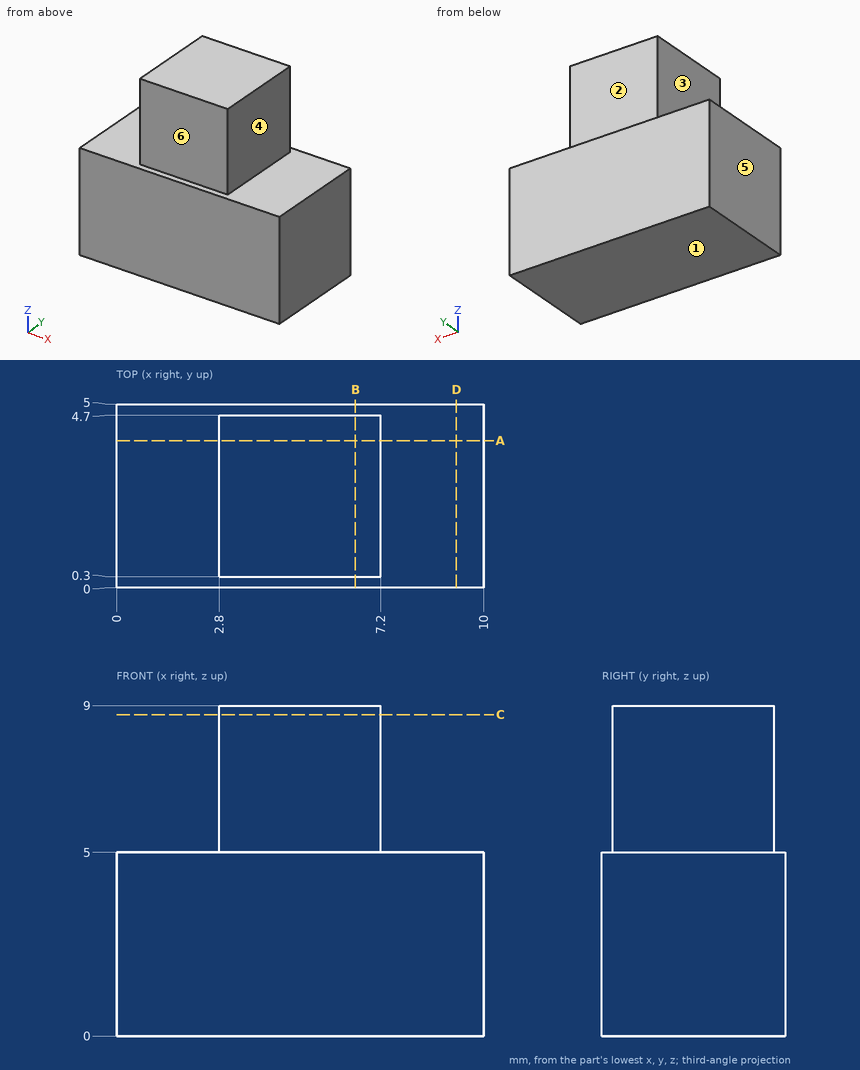
Geometry check sheet. Reference: drawing and pictorial views, mm from the part's lowest x, y, z. A direction names the side the tool comes from. Coordinates: 2 decimals unless noted, no trailing zeros. Loops run counter-clockwise (first coordinate to the right, second up) from the corner with the lowest first, then second, coordinate; pieces in that order, holes last. Notation, with made-up numbers: (66, 0.25) -> (106, 0.25) arc R17 ccw to (106, 30.25) -> close; hole circle Ø10 at (37.25, 33). An arc over 180 degrees is marked (long way). Write item = value, one per line. Start each with the question number.
1. Depth check by flat-ended pin: P1, Ø2, axis at y = 3.5, z = 6.5, coming from the +X side; P2, Ø2, axis at y = 1.5, z = 6.5, coming from the -X side; P3, Ø3, axis at x = 1, y = 4.5, coming from the +Z side. Enter the tip coordinate at first touch or a pass-through.
2. Section check A-A on y = 4. Record the cut outline in (x, z), then the cut area to 3 significant figures.
3. Section check C-C on z = 8.75. Record the cut outline in (x, y), then the cut area to 3 significant figures.
4. Tool access check on the marked faces 1, 2 and 3. Record the directions out of +Z, -Z, +X, -X, +Y, -Y that give a thin tool (end or side, any length) a straight path to the whole face; none if there is none.
5. Draft check along X on the marked faces 4, 5 and 6. Enter one of: released by +X, released by -X, zero draft, split by the parting line, or undercut.
6. Section check D-D on x = 9.25. Record the cut outline in (y, z).
7. Material ranges on line 1 (X direction, y = 0.65, z = 6.5); line 2 (Y direction, x = 6.25, z = 8); line 3 (Z direction, x = 1.75, y = 0.7), recorded low to high.
8. Section check B-B on x = 6.5. Record the cut outline in (y, z), then the cut area to 3 significant figures.
Responses:
q1.P1 = 7.2
q1.P2 = 2.8
q1.P3 = 5
q2.outline = (0, 0) -> (10, 0) -> (10, 5) -> (7.2, 5) -> (7.2, 9) -> (2.8, 9) -> (2.8, 5) -> (0, 5) -> close
q2.area = 67.6 mm2
q3.outline = (2.8, 0.3) -> (7.2, 0.3) -> (7.2, 4.7) -> (2.8, 4.7) -> close
q3.area = 19.4 mm2
q4.face_1 = -Z, +X, -X, +Y, -Y
q4.face_2 = +Z, +X, -X, +Y
q4.face_3 = +Z, -X, +Y, -Y
q5.face_4 = released by +X
q5.face_5 = released by -X
q5.face_6 = zero draft
q6.outline = (0, 0) -> (5, 0) -> (5, 5) -> (0, 5) -> close
q7.line_1 = 2.8 to 7.2
q7.line_2 = 0.3 to 4.7
q7.line_3 = 0 to 5
q8.outline = (0, 0) -> (5, 0) -> (5, 5) -> (4.7, 5) -> (4.7, 9) -> (0.3, 9) -> (0.3, 5) -> (0, 5) -> close
q8.area = 42.6 mm2
